from build123d import *

# Parameters (mm, degrees)
SKETCH1_W           = 292.1
SKETCH1_H           = 165.1
BOSS_EXTRUDE1_DEPTH = 6.35
CUT_EXTRUDE1_DEPTH  = 168.885161643


with BuildPart() as part:
    # Sketch1 → Boss-Extrude1 (new body)
    with BuildSketch(Plane.XY):
        Rectangle(SKETCH1_W, SKETCH1_H)
    extrude(amount=BOSS_EXTRUDE1_DEPTH)

    # Sketch2 → Cut-Extrude1 (cut, through all)
    with BuildSketch(Plane.XY.offset(6.35)):
        with BuildLine():
            Line((-146.05, 52.07), (-88.9, 52.07))
            ThreePointArc((-88.9, 52.07), (-84.409871939, 50.210128061), (-82.55, 45.72))
            Line((-82.55, 45.72), (-82.55, 20.32))
            ThreePointArc((-82.55, 20.32), (-84.409871939, 15.829871939), (-88.9, 13.97))
            Line((-88.9, 13.97), (-146.05, 13.97))
            Line((-146.05, 13.97), (-146.05, 52.07))
        make_face()
        with BuildLine():
            Line((-146.05, -13.97), (-146.05, -52.07))
            Line((-146.05, -52.07), (-88.9, -52.07))
            ThreePointArc((-88.9, -52.07), (-84.409871939, -50.210128061), (-82.55, -45.72))
            Line((-82.55, -45.72), (-82.55, -20.32))
            ThreePointArc((-82.55, -20.32), (-84.409871939, -15.829871939), (-88.9, -13.97))
            Line((-88.9, -13.97), (-146.05, -13.97))
        make_face()
        with BuildLine():
            Line((146.05, -52.07), (88.9, -52.07))
            ThreePointArc((88.9, -52.07), (84.409871939, -50.210128061), (82.55, -45.72))
            Line((82.55, -45.72), (82.55, -20.32))
            ThreePointArc((82.55, -20.32), (84.409871939, -15.829871939), (88.9, -13.97))
            Line((88.9, -13.97), (146.05, -13.97))
            Line((146.05, -13.97), (146.05, -52.07))
        make_face()
        with BuildLine():
            Line((146.05, 13.97), (146.05, 52.07))
            Line((146.05, 52.07), (88.9, 52.07))
            ThreePointArc((88.9, 52.07), (84.409871939, 50.210128061), (82.55, 45.72))
            Line((82.55, 45.72), (82.55, 20.32))
            ThreePointArc((82.55, 20.32), (84.409871939, 15.829871939), (88.9, 13.97))
            Line((88.9, 13.97), (146.05, 13.97))
        make_face()
    extrude(amount=-CUT_EXTRUDE1_DEPTH, mode=Mode.SUBTRACT)


solid = part.part
CAD build for the part. Positions are in the model's coordinates, mm. A direction names the side the tool comes from. Give positions to 0.01 mm unless a question says otherwise; leave off trailing zeros. Loops run counter-clockwise (first coordinate to the right, second up) from the corner with the lowest first, then second, coordinate; pieces in that order, holes last. Notation, with made-up numbers: M 71,23 L 76,23 A14 ccw 76,29 Z; hole C -21,22 d5. An arc over 180 degrees is marked long. Write each question's results on one line, items separated by ' | '.
Q1. Probe probe 1 along Y at (x, z) = (-115.5, 2); probe 2 along X at (y, z) = (-37.5, 4.5); probe 3 along X at (y, z) = (50.5, 4.75). List the from-to ranges inside material, lowest first.
Geometry check:
probe 1: y = -82.55 to -52.07, -13.97 to 13.97, 52.07 to 82.55 | probe 2: x = -82.55 to 82.55 | probe 3: x = -84.72 to 84.72
Q2. Band-saw the part on A-A on x = -101. Write the cut outline in (y, z).
Geometry check:
outline: M -82.55,0 L -52.07,0 L -52.07,6.35 L -82.55,6.35 Z; M -13.97,0 L 13.97,0 L 13.97,6.35 L -13.97,6.35 Z; M 52.07,0 L 82.55,0 L 82.55,6.35 L 52.07,6.35 Z
Q3. Mould opens along Y. For faces 1 (the face through (-2, -82.55, 3)), 2 (the face through (-2, 1, 0)), 3 (the face through (118, 52.07, 3)), 4 (the face through (84.5, 50.3, 3.2)) say: pulls with the +Y half, pulls with the -Y half, needs draft (parallel to the pull), parting line crosses it, or undercut.
Geometry check:
face 1: pulls with the -Y half | face 2: needs draft | face 3: undercut | face 4: undercut
Q4. Band-saw the part on D-D on y = 49. Write the cut outline in (x, z), and give its area (3 significant figures).
Geometry check:
outline: M -83.46,0 L 83.46,0 L 83.46,6.35 L -83.46,6.35 Z | area: 1,060 mm²
Q5. Band-saw the part on B-B on z = 1. Write the cut outline in (x, y).
Geometry check:
outline: M -146.05,-82.55 L 146.05,-82.55 L 146.05,-52.07 L 88.9,-52.07 A6.35 cw 82.55,-45.72 L 82.55,-20.32 A6.35 cw 88.9,-13.97 L 146.05,-13.97 L 146.05,13.97 L 88.9,13.97 A6.35 cw 82.55,20.32 L 82.55,45.72 A6.35 cw 88.9,52.07 L 146.05,52.07 L 146.05,82.55 L -146.05,82.55 L -146.05,52.07 L -88.9,52.07 A6.35 cw -82.55,45.72 L -82.55,20.32 A6.35 cw -88.9,13.97 L -146.05,13.97 L -146.05,-13.97 L -88.9,-13.97 A6.35 cw -82.55,-20.32 L -82.55,-45.72 A6.35 cw -88.9,-52.07 L -146.05,-52.07 Z
Q6. Band-saw the part on C-C on y = -28.5. Write the cut outline in (x, z), and give its area (3 significant figures).
Geometry check:
outline: M -82.55,0 L 82.55,0 L 82.55,6.35 L -82.55,6.35 Z | area: 1,050 mm²
Q7. Which spindle directions (+Z, -Z, +X, -X, +Y, -Y) get a long thin tool onto all of the face, cutting with end or side? Do faces 5 (the face through (-2, 1, 6.35)), 6 (the face through (-84.36, -15.88, 3.22)), 7 (the face through (117, 13.97, 3)). Say none if no direction does.
Geometry check:
face 5: +Z, +X, -X, +Y, -Y | face 6: +Z, -Z, -X | face 7: +Z, -Z, +X
Q8. Flat gauge pin, fed straight in: P1, Ø2, axis at y = -32.5, z = 3.5, coming from the -X side. Where does the tip first touch, or does it go through?
Geometry check:
P1: stops at x = -82.55
